```python
from build123d import *

# Parameters (mm, degrees)
ESQUISSE1_R             = 5
BOSS_EXTRU_1_DEPTH      = 6
BOSS_EXTRU_2_DEPTH      = 5
BOSS_EXTRU_2_DEPTH_BACK = 1
ESQUISSE2_R             = 2.5
ESQUISSE3_R             = 1.5
ENL_V_MAT_EXTRU_2_DEPTH = 6
ESQUISSE4_R             = 2.55
ENL_V_MAT_EXTRU_3_DEPTH = 5


with BuildPart() as part:
    # Esquisse1 → Boss.-Extru.1 (new body)
    with BuildSketch(Plane(origin=(0, 0, 0), x_dir=(1, 0, 0), z_dir=(0, 1, 0))):
        with Locations(Location((0, 0, 0), (0, 0, 270))):
            Circle(ESQUISSE1_R)
    extrude(amount=BOSS_EXTRU_1_DEPTH)

    # Esquisse2 → Boss.-Extru.2 (add, two sides: drawn at the far end of the back side and taken through both)
    with BuildSketch(Plane(origin=(0, 6, 0), x_dir=(1, 0, 0), z_dir=(0, 1, 0)).offset(-BOSS_EXTRU_2_DEPTH_BACK)):
        with Locations(Location((0, 0, 0), (0, 0, 270))):
            Circle(ESQUISSE2_R)
    extrude(amount=BOSS_EXTRU_2_DEPTH + BOSS_EXTRU_2_DEPTH_BACK)

    # Esquisse3 → Enlèv. mat.-Extru.2 (cut)
    with BuildSketch(Plane(origin=(0, 11, 0), x_dir=(1, 0, 0), z_dir=(0, 1, 0))):
        with Locations(Location((0, 0, 0), (0, 0, 270))):
            Circle(ESQUISSE3_R)
    extrude(amount=-ENL_V_MAT_EXTRU_2_DEPTH, mode=Mode.SUBTRACT)

    # Esquisse4 → Enlèv. mat.-Extru.3 (cut)
    with BuildSketch(Plane.XZ):
        with Locations(Location((0, 0, 0), (0, 0, 270))):
            Circle(ESQUISSE4_R)
    extrude(amount=-ENL_V_MAT_EXTRU_3_DEPTH, mode=Mode.SUBTRACT)


solid = part.part
```
The listing builds one solid part. Answer for the finished solid, in the listing's coordinates (mm). A direction names the side the tool comes from. Coordinates: 2 decimals unless noted, no trailing zeros. Write each loop counter-clockwise with the first axis right and the second up, starting at its lowest first coordinate (ties: lowest second). Pieces come first, ordered by that corner, then holes. Notation, with made-up numbers: (24.25, -1) - (48.25, -1) arc R18 ccw to (48.25, 17) - close; hole circle Ø3 at (32.25, 21). An arc over 180 degrees is marked (long way). One line per item, written item: value.
1) Consider line 1 along X through (y, z) = (9.7, 0); line 2 along X through (y, z) = (1.2, 0); line 3 along Y through (x, z) = (-1.5, -3.5). Determine where each line is inside the solid, lowest interval first. Write a range as from..to.
Geometry check:
line 1: x = -2.5..-1.5, 1.5..2.5
line 2: x = -5..-2.55, 2.55..5
line 3: y = 0..6
2) A tool of negligible diameter and unlimited length cuts with its end or side. For faces 1 (the cylindrical face through (-2.44, 8.46, -0.54)), 2 (the flat face through (-2, 0, 2)), 3 (the flat face through (0, 5, -2)), from which of +Z, -Z, +X, -X, +Y, -Y can it reach the whole face along a straight path? Write none if from no direction.
Geometry check:
face 1: +Y
face 2: +Z, -Z, +X, -X, -Y
face 3: -Y
3) For a pull along X with two mould halves and no side action, classify faces 4 (the flat face through (-2, 11, 0)), 5 (the cylindrical face through (0.45, 8.04, 1.43)), 6 (the cylindrical face through (-4.88, 2.96, -1.08)) as pulls with the +X half, pulls with the -X half, needs draft (parallel to the pull), parting line crosses it, or undercut.
Geometry check:
face 4: needs draft
face 5: undercut
face 6: parting line crosses it
4) Find section B-B (z = 0). Give the vertices of the cut face in (x, y).
Geometry check:
outline: (-5, 0) - (-2.55, 0) - (-2.55, 5) - (-1.5, 5) - (-1.5, 11) - (-2.5, 11) - (-2.5, 6) - (-5, 6) - close; (1.5, 5) - (2.55, 5) - (2.55, 0) - (5, 0) - (5, 6) - (2.5, 6) - (2.5, 11) - (1.5, 11) - close
5) Each of these flat-tipped pins is pushed along its axis until it touches: pin 1 Ø5 at (x, z) = (0.5, -0.5) entering from +Y; pin 2 Ø1.5 at (y, z) = (5.5, 1) entering from -X; pin 3 Ø2.5 at (x, z) = (1, 0) entering from -Y; pin 4 Ø4 at (x, y) = (2.5, 2.5) entering from +Z. Where does it stop, or does it pass through?
Geometry check:
pin 1: stops at y = 11
pin 2: stops at x = -4.99
pin 3: stops at y = 5
pin 4: stops at z = 4.97
6) Find section C-C (y = 9.75). Give the vertices of the cut face in (x, z).
Geometry check:
outline: circle Ø5 at (0, 0); hole circle Ø3 at (0, 0)
7) Find section D-D (z = 2). Give the vertices of the cut face in (x, y).
Geometry check:
outline: (-4.58, 0) - (-1.58, 0) - (-1.58, 5) - (1.58, 5) - (1.58, 0) - (4.58, 0) - (4.58, 6) - (1.5, 6) - (1.5, 11) - (-1.5, 11) - (-1.5, 6) - (-4.58, 6) - close
8) Find section A-A (x = 0). Give the vertices of the cut face in (y, z).
Geometry check:
outline: (0, -5) - (6, -5) - (6, -2.5) - (11, -2.5) - (11, -1.5) - (5, -1.5) - (5, -2.55) - (0, -2.55) - close; (0, 2.55) - (5, 2.55) - (5, 1.5) - (11, 1.5) - (11, 2.5) - (6, 2.5) - (6, 5) - (0, 5) - close
